```python
from build123d import *

# Parameters (mm, degrees)
SKETCH2_R                = 17.5
SKETCH2_R_2              = 5
BOSS_EXTRUDE1_DEPTH      = 25
CUT_EXTRUDE1_START       = -9
SKETCH3_R                = 15
SKETCH3_R_2              = 5
CUT_EXTRUDE1_DEPTH       = 9
BOSS_EXTRUDE2_REACH      = 82.971
BOSS_EXTRUDE2_END_RADIUS = 17.5
SKETCH5_R                = 17.5
SKETCH5_R_2              = 5
SKETCH6_R                = 15
SKETCH6_R_2              = 5
CUT_EXTRUDE2_DEPTH       = 9


with BuildPart() as part:
    # Sketch2 → Boss-Extrude1 (new, symmetric)
    with BuildSketch(Plane(origin=(0, 0, 0), x_dir=(0, 0, -1), z_dir=(1, 0, 0))):
        Circle(SKETCH2_R)
        Circle(SKETCH2_R_2, mode=Mode.SUBTRACT)
    extrude(amount=BOSS_EXTRUDE1_DEPTH, both=True)

    # Sketch3 → Cut-Extrude1 (cut)
    with BuildSketch(Plane(origin=(25, 0, 0), x_dir=(0, 0, -1), z_dir=(1, 0, 0)).offset(CUT_EXTRUDE1_START)):
        Circle(SKETCH3_R)
        Circle(SKETCH3_R_2, mode=Mode.SUBTRACT)
    cut_extrude1 = extrude(amount=CUT_EXTRUDE1_DEPTH, mode=Mode.SUBTRACT)

    # Mirror1: Cut-Extrude1 across plane
    add(cut_extrude1.mirror(Plane(origin=(0, 0, 0), x_dir=(0, 0, 1), z_dir=(1, 0, 0))), mode=Mode.SUBTRACT)

    # Boss-Extrude2: up to this cylinder (the profile starts outside it)
    boss_extrude2_end = Plane(origin=(0, 0, 0), z_dir=(-1, 0, 0)) * Cylinder(BOSS_EXTRUDE2_END_RADIUS, 201.942, mode=Mode.PRIVATE)
    # Sketch5 → Boss-Extrude2 (add, up to the surface)
    with BuildSketch(Plane(origin=(0, 57.5, 0), x_dir=(1, 0, 0), z_dir=(0, 1, 0)), mode=Mode.PRIVATE) as boss_extrude2_sk1:
        with Locations(Location((0, 0, 0), (0, 0, 270))):
            Circle(SKETCH5_R)
        with Locations(Location((0, 0, 0), (0, 0, 270))):
            Circle(SKETCH5_R_2, mode=Mode.SUBTRACT)
    boss_extrude2_tool1 = extrude(boss_extrude2_sk1.sketch, amount=-BOSS_EXTRUDE2_REACH, mode=Mode.PRIVATE) - boss_extrude2_end
    add(boss_extrude2_tool1.solids().sort_by_distance((0, 57.5, -17.005025))[0])

    # Sketch6 → Cut-Extrude2 (cut)
    with BuildSketch(Plane(origin=(0, 57.5, 0), x_dir=(1, 0, 0), z_dir=(0, 1, 0))):
        with Locations(Location((0, 0, 0), (0, 0, 270))):
            Circle(SKETCH6_R)
        with Locations(Location((0, 0, 0), (0, 0, 270))):
            Circle(SKETCH6_R_2, mode=Mode.SUBTRACT)
    extrude(amount=-CUT_EXTRUDE2_DEPTH, mode=Mode.SUBTRACT)


solid = part.part
```
Source: CAD feature listing. Evaluate the final solid. Frame: model axes, mm. A direction names the side the tool comes from. Round coordinates to 2 decimals unless told otherwise and drop trailing zeros. Loops run counter-clockwise (first coordinate to the right, second up) from the corner with the lowest first, then second, coordinate; pieces in that order, holes last. Notation, with made-up numbers: (81, 5.25) - (120, 5.25) arc R19 ccw to (120, 13.25) - close; hole circle Ø4 at (55.25, 7.5). An arc over 180 degrees is marked (long way). Use CSV: the item, a comma, the result in double quotes.
Q1. Reachability of faces 5 (the cylindrical face through (-20.437, 0.66, 14.985)), 6 (the flat face through (16, 4, 4)), 7 (the cylindrical face through (-0.22, -4.88, 1.08)), 8 (the flat face through (4, 48.5, -4)), 9 (the flat face through (25, 8, -13)) from +Z, -Z, +X, -X, +Y, -Y: full face, straight path, thin tool, end or side. Return the list, or none.
Reported:
face 5,"-X"
face 6,"+X"
face 7,"+X, -X"
face 8,"+Y"
face 9,"+Z, -Z, +X, +Y, -Y"
Q2. Mould query, pull axis Y, two halves, no side actions, for faces 1 (the cylindrical face through (0.35, -17.084, 3.794)), 2 (the cylindrical face through (20.437, 0.66, 14.985)), 3 (the flat face through (-25, 8, -13)), 4 (the flat face through (8, 57.5, 13)). Classes: pulls with the +Y half, pulls with the -Y half, needs draft (parallel to the pull), parting line crosses it, or undercut.
Reported:
face 1,"parting line crosses it"
face 2,"undercut"
face 3,"needs draft"
face 4,"pulls with the +Y half"
Q3. Section query A-A, the plane z = 0. Output: boundary loops of the cut face in (x, y).
Reported:
outline,"(-25, -17.5) - (25, -17.5) - (25, -15) - (16, -15) - (16, -5) - (-16, -5) - (-16, -15) - (-25, -15) - close; (-25, 15) - (-16, 15) - (-16, 5) - (16, 5) - (16, 15) - (25, 15) - (25, 17.5) - (17.5, 17.5) - (17.5, 57.5) - (15, 57.5) - (15, 48.5) - (5, 48.5) - (5, 17.5) - (-5, 17.5) - (-5, 48.5) - (-15, 48.5) - (-15, 57.5) - (-17.5, 57.5) - (-17.5, 17.5) - (-25, 17.5) - close"
Q4. Section query C-C, the plane y = 26. Output: boundary loops of the cut face in (x, z).
Reported:
outline,"circle Ø35 at (0, 0); hole circle Ø10 at (0, 0)"
Q5. Pin query (flat end, axial travel): pin 1 Ø5 at (x, y) = (-0.5, 44) entering from -Z; pin 2 Ø15 at (y, z) = (0.5, -0.5) entering from -X; pin 3 Ø3 at (x, y) = (-18, 13.5) entering from +Z; pin 4 Ø3 at (x, y) = (8.5, 35) entering from -Z. Return the tip coordinate at first contact, or that it passes through.
Reported:
pin 1,"z = -17.5"
pin 2,"x = -16"
pin 3,"z = 12.74"
pin 4,"z = -16.04"
Q6. Ray query, line 1 along X through (y, z) = (44.5, 0); line 2 along Y through (x, z) = (22.25, 0); line 3 along X through (y, z) = (-2.5, 5.5). Return the intervals inside material, ascending.
Reported:
line 1,"-17.5 to -5, 5 to 17.5"
line 2,"-17.5 to -15, 15 to 17.5"
line 3,"-16 to 16"
Q7. Section query B-B, the plane x = 0. Output: boundary loops of the cut face in (y, z), then the cut area to 3 significant figures.
Reported:
outline,"(0, -17.5) - (57.5, -17.5) - (57.5, -15) - (48.5, -15) - (48.5, -5) - (16.77, -5) arc R17.5 ccw to (16.77, 5) - (48.5, 5) - (48.5, 15) - (57.5, 15) - (57.5, 17.5) - (0, 17.5) arc R17.5 ccw to start; hole circle Ø10 at (0, 0)"
area,"1,830 mm^2"
Q8. Section query D-D, the plane y = 14. Output: boundary loops of the cut face in (x, z), then the cut area to 3 significant figures.
Reported:
outline,"(-25, -10.5) - (-14, -10.5) arc R17.5 ccw to (14, -10.5) - (25, -10.5) - (25, -5.39) - (16, -5.39) - (16, 5.39) - (25, 5.39) - (25, 10.5) - (14, 10.5) arc R17.5 ccw to (-14, 10.5) - (-25, 10.5) - (-25, 5.39) - (-16, 5.39) - (-16, -5.39) - (-25, -5.39) - close"
area,"1,130 mm^2"
